```python
from build123d import *

# Parameters (mm, degrees)
SKETCH_1_R          = 19
SKETCH_1_R_2        = 2
SKETCH_1_R_3        = 7.5
SKETCH_1_R_4        = 1.6
EXTRUDE_1_DEPTH     = 5.6
SKETCH_2_W          = 15.17824661
SKETCH_2_H          = 4
CUT_EXTRUDE_1_DEPTH = 10
FILLET_1_R          = 1
CHAMFER_1_SIZE      = 0.5
CHAMFER_2_SIZE      = 0.5


with BuildPart() as part:
    # 草图1 → 凸台-拉伸1 (new body)
    with BuildSketch(Plane(origin=(0, 0, 0), x_dir=(1, 0, 0), z_dir=(0, 1, 0))):
        with Locations(Location((0, 0, 0), (0, 0, 270))):
            Circle(SKETCH_1_R)
        with Locations(Location((0, -12.15, 0), (0, 0, 270))):
            Circle(SKETCH_1_R_2, mode=Mode.SUBTRACT)
        with Locations(Location((10.522208656, 6.075, 0), (0, 0, 270))):
            Circle(SKETCH_1_R_2, mode=Mode.SUBTRACT)
        with Locations(Location((-10.522208656, 6.075, 0), (0, 0, 270))):
            Circle(SKETCH_1_R_2, mode=Mode.SUBTRACT)
        with Locations(Location((0, 0, 0), (0, 0, 270))):
            Circle(SKETCH_1_R_3, mode=Mode.SUBTRACT)
        with Locations(Location((-11.691342951, -6.75, 0), (0, 0, 270))):
            Circle(SKETCH_1_R_4, mode=Mode.SUBTRACT)
        with Locations(Location((11.691342951, -6.75, 0), (0, 0, 270))):
            Circle(SKETCH_1_R_4, mode=Mode.SUBTRACT)
        with Locations(Location((0, 13.5, 0), (0, 0, 270))):
            Circle(SKETCH_1_R_4, mode=Mode.SUBTRACT)
    extrude(amount=EXTRUDE_1_DEPTH)

    # 草图2 → 切除-拉伸1 (cut)
    with BuildSketch(Plane(origin=(0, 5.6, 0), x_dir=(1, 0, 0), z_dir=(0, 1, 0))):
        with Locations((19.589123305, 0)):
            Rectangle(SKETCH_2_W, SKETCH_2_H)
    extrude(amount=-CUT_EXTRUDE_1_DEPTH, mode=Mode.SUBTRACT)

    # 圆角1
    fillet_1_edges = [part.edges().sort_by_distance(p)[0] for p in [
        (12, 2.8, 2),
        (18.894443628, 2.8, -2),
        (12, 2.8, -2),
        (18.894443628, 2.8, 2),
    ]]
    fillet(fillet_1_edges, radius=FILLET_1_R)

    # 倒角1
    chamfer_1_edges = [part.edges().sort_by_distance(p)[0] for p in [
        (-19, 5.6, 0),
        (-19, 0, 0),
        (15.374119675, 5.6, -2),
        (15.374119675, 5.6, 2),
        (12, 5.6, 0),
        (18.512001965, 5.6, -2.354502776),
        (18.512001965, 5.6, 2.354502776),
        (15.374119675, 0, 2),
        (15.374119675, 0, -2),
        (12, 0, 0),
        (18.512001965, 0, -2.354502776),
        (18.512001965, 0, 2.354502776),
        (12.292893219, 5.6, 1.707106781),
        (12.292893219, 0, 1.707106781),
        (12.292893219, 5.6, -1.707106781),
        (12.292893219, 0, -1.707106781),
    ]]
    chamfer(chamfer_1_edges, length=CHAMFER_1_SIZE)

    # 倒角2
    chamfer_2_edges = [part.edges().sort_by_distance(p)[0] for p in [
        (0, 5.6, 10.15),
        (0, 0, -15.1),
        (11.691342951, 0, 5.15),
        (-11.691342951, 0, 5.15),
        (0, 0, -7.5),
        (-10.522208656, 0, -8.075),
        (10.522208656, 0, -8.075),
        (0, 0, 10.15),
        (10.522208656, 5.6, -8.075),
        (-10.522208656, 5.6, -8.075),
        (0, 5.6, -7.5),
        (-11.691342951, 5.6, 5.15),
        (11.691342951, 5.6, 5.15),
        (0, 5.6, -15.1),
    ]]
    chamfer(chamfer_2_edges, length=CHAMFER_2_SIZE)


solid = part.part
```
Geometry: final body of the model. Coordinates: model frame, mm. A direction names the side the tool comes from. Round coordinates to 2 decimals unless told otherwise and drop trailing zeros. Loops run counter-clockwise (first coordinate to the right, second up) from the corner with the lowest first, then second, coordinate; pieces in that order, holes last. Notation, with made-up numbers: (77, 85.25) -> (104, 85.25) arc R10 ccw to (104, 92.25) -> close; hole circle Ø1 at (54, 65.5). An arc over 180 degrees is marked (long way). Use one line per item in the form item = value.
Item 1: Draft query along Z for faces 5 (the flat face through (-8, 0, 4)), 6 (the cylindrical face through (-18.984, 2.768, -0.791)), 7 (the flat face through (15, 3, 2)). Return one class per face: released by +Z, released by -Z, zero draft, split by the parting line, or undercut.
Evaluation:
face_5 = zero draft
face_6 = split by the parting line
face_7 = undercut
Item 2: Material intervals for probe 1 along Z at (x, y) = (13, 4.45); probe 2 along Z at (x, y) = (-11.5, 0.45); probe 3 along Z at (x, y) = (-10, 1.75), sorted ascending.
Evaluation:
probe_1 = -13.86 to -2, 2 to 5.83, 7.67 to 13.86
probe_2 = -15.06 to -7.88, -4.27 to 5.11, 8.39 to 15.06
probe_3 = -16.16 to -8.01, -4.14 to 16.16
Item 3: Access query for faces 1 (the conical face through (12.16, 5.3, -1.86)), 2 (the cylindrical face through (13.278, 2.768, 6.542)), 3 (the cylindrical face through (12.285, 2.768, -1.699)), 4 (the conical face through (12.16, 0.3, 1.86)). Directions: +Z, -Z, +X, -X, +Y, -Y. A direction counts if a zero-diameter tool reaches every point of the face in a straight line with its end or side. Return the directions, or none.
Evaluation:
face_1 = +X, +Y
face_2 = +Y, -Y
face_3 = +X, +Y, -Y
face_4 = +X, -Y
Item 4: Cut plane C-C on y = 2.7. Output: boundary loops of the cut face in (x, z) (3 decimals), then the cut area to 3 significant figures.
Evaluation:
outline = (12, -1) -> (12, 1) arc R1 cw to (13, 2) -> (17.748, 2) arc R1 ccw to (18.734, 3.167) arc R19 ccw (long way) to (18.734, -3.167) arc R1 ccw to (17.748, -2) -> (13, -2) arc R1 cw to start; hole circle Ø3.2 at (-11.691, 6.75); hole circle Ø4 at (-10.522, -6.075); hole circle Ø15 at (0, 0); hole circle Ø4 at (0, 12.15); hole circle Ø3.2 at (0, -13.5); hole circle Ø4 at (10.522, -6.075); hole circle Ø3.2 at (11.691, 6.75)
area = 868 mm2
Item 5: Contact query for flat-ended pins moving along their axis: pin 1 Ø12 at (x, z) = (0, 0) entering from -Y; pin 2 Ø0.6 at (y, z) = (2.5, -0.5) entering from +X; pin 3 Ø2.5 at (x, y) = (14.5, 2.5) entering from +Z; pin 4 Ø3.5 at (x, z) = (-11.69, 6.75) entering from -Y. Output: stop coordinate, or through.
Evaluation:
pin_1 = through
pin_2 = 12
pin_3 = 13.62
pin_4 = 0.35
Item 6: Cut plane A-A on x = 0. Give the number of separate pieces and of enclosed holes in the cut face, then the cut area to 3 significant figures.
Evaluation:
separate_pieces = 4
enclosed_holes = 0
area = 86.5 mm2
Item 7: Cut plane B-B on z = 0. Output: boundary loops of the cut face in (x, y), then the cut area to 3 significant figures.
Evaluation:
outline = (-19, 0.5) -> (-18.5, 0) -> (-8, 0) -> (-7.5, 0.5) -> (-7.5, 5.1) -> (-8, 5.6) -> (-18.5, 5.6) -> (-19, 5.1) -> close; (7.5, 0.5) -> (8, 0) -> (11.5, 0) -> (12, 0.5) -> (12, 5.1) -> (11.5, 5.6) -> (8, 5.6) -> (7.5, 5.1) -> close
area = 88.6 mm2
